For this review, take the finished solid that the model builds, in its own axes (mm). A direction names the side the tool comes from. Coordinates: 2 decimals unless noted, no trailing zeros. Loops run counter-clockwise (first coordinate to the right, second up) from the corner with the lowest first, then second, coordinate; pieces in that order, holes last. Notation, with made-up numbers: (29.25, 68.5) -> (59.25, 68.5) arc R34 cw to (59.25, 101.5) -> close; hole circle Ø1 at (-6, 20.25). An arc over 180 degrees is marked (long way). Use a Markdown table: item, result.
from build123d import *

# Parameters (mm, degrees)
SKETCH1_W           = 5
SKETCH1_H           = 9.685479934
BOSS_EXTRUDE1_DEPTH = 5


with BuildPart() as part:
    # Sketch1 → Boss-Extrude1 (new body)
    with BuildSketch(Plane.XY):
        Polygon((100, 30), (100, 47.229662795), (0, 25), (0, 0), (100, 0), (100, 10), (115, 10), (115, 30), align=None)
        with Locations((107.5, 19.842739967)):
            Rectangle(SKETCH1_W, SKETCH1_H, mode=Mode.SUBTRACT)
    extrude(amount=BOSS_EXTRUDE1_DEPTH)


solid = part.part
(1) For line 1 along Y through (x, z) = (107.5, 3.25); line 2 along X through (y, z) = (15.5, 3.1); line 3 along Y through (x, z) = (101.5, 1.55), list the stretches that pass through material, from the lowest coordinate up.
Found:
| item | result |
|---|---|
| line 1 | y = 10 to 15, 24.69 to 30 |
| line 2 | x = 0 to 105, 110 to 115 |
| line 3 | y = 10 to 30 |
(2) For faces 4 (the face through (107, 24.685, 2)), 5 (the face through (57, 19, 5)), 6 (the face through (107, 10, 2)), 7 (the face through (108, 30, 2)), list the 3-axis set-ups (+Z, -Z, +X, -X, +Y, -Y) from which the entire face can be reached by the end or side of a thin tool; tool diameter is ignored.
Found:
| item | result |
|---|---|
| face 4 | +Z, -Z |
| face 5 | +Z, +X, -X, +Y, -Y |
| face 6 | +Z, -Z, +X, -Y |
| face 7 | +Z, -Z, +X, +Y |
(3) Take a section at D-D on x = 86. Write out the cut boundary in (y, z).
Found:
| item | result |
|---|---|
| outline | (0, 0) -> (44.12, 0) -> (44.12, 5) -> (0, 5) -> close |
(4) Take a section at C-C on y = 4. Write out the cut boundary in (x, z), plus the area to 3 significant figures.
Found:
| item | result |
|---|---|
| outline | (0, 0) -> (100, 0) -> (100, 5) -> (0, 5) -> close |
| area | 500 mm^2 |
(5) Mouldability with a two-part tool opening along X and no side actions: class faces 1 (the face through (100, 5, 2)), 2 (the face through (107, 15, 2)), 3 (the face through (57, 19, 0)) as pulls with the +X half, pulls with the -X half, needs draft (parallel to the pull), parting line crosses it, or undercut.
Found:
| item | result |
|---|---|
| face 1 | pulls with the +X half |
| face 2 | undercut |
| face 3 | needs draft |
(6) Take a section at B-B on z = 1.45. Write out the cut boundary in (x, y), plus the area to 3 significant figures.
Found:
| item | result |
|---|---|
| outline | (0, 0) -> (100, 0) -> (100, 10) -> (115, 10) -> (115, 30) -> (100, 30) -> (100, 47.23) -> (0, 25) -> close; hole (105, 15) -> (110, 15) -> (110, 24.69) -> (105, 24.69) -> close |
| area | 3,860 mm^2 |
(7) For pin 1 Ø3 at (x, z) = (23, 4) entering from +Y; pin 2 Ø1.5 at (x, z) = (106.5, 1.5) entering from +Y, all flat-tipped, find the tip position at first contact; note any pin that passes through.
Found:
| item | result |
|---|---|
| pin 1 | stops at y = 30.45 |
| pin 2 | stops at y = 30 |
(8) Take a section at A-A on y = 18. Write out the cut boundary in (x, z), plus the area to 3 significant figures.
Found:
| item | result |
|---|---|
| outline | (0, 0) -> (105, 0) -> (105, 5) -> (0, 5) -> close; (110, 0) -> (115, 0) -> (115, 5) -> (110, 5) -> close |
| area | 550 mm^2 |
